Read the model definition and answer for the solid it produces. Units are mm, in the model's axes. Give positions to 0.01 mm unless a question says otherwise; leave off trailing zeros. Write each loop counter-clockwise with the first axis right and the second up, starting at its lowest first coordinate (ties: lowest second). Pieces come first, ordered by that corner, then holes. Notation, with made-up numbers: M 26.5,32.25 L 70.5,32.25 A30 ccw 70.5,70.25 Z; hole C -28.75,77.5 d8. An arc over 180 degrees is marked long. Use a Markdown table: item, result. Add a question column.
Item 1: A cutting plane is placed at A-A on x = 29. Determine the outline of the cut face in (y, z), then the cut area to 3 significant figures.
Item 2: A cutting plane is placed at D-D on z = 14.25. Determine the outline of the cut face in (x, y).
Item 3: Consider probe 1 along X at (y, z) = (66, 2.5); probe 2 along Z at (x, y) = (23.5, 40); probe 3 along X at (y, z) = (47, 3). Determine where each line is inside the solid, lowest interval first. Write a range as [from, to].
Item 4: A cutting plane is placed at C-C on x = 19. Determine the outline of the cut face in (y, z), then the cut area to 3 significant figures.
Item 5: Given P1, Ø1, axis at x = 13.5, y = 51, coming from the +Z side; P2, Ø9.5, axis at x = 21.5, y = 54, coming from the +Z side; P3, Ø8, axis at x = 26, z = 7.5, coming from the -Y side, each flat-ended and moving along its own axis, determine where each tip first touches the part or whether it passes through.
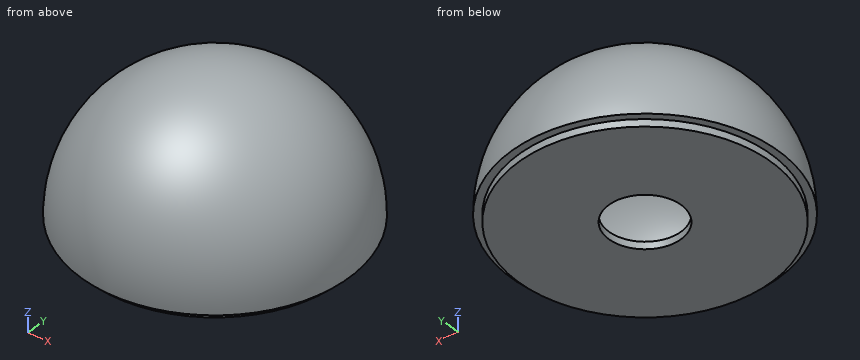
Autodesk Inventor part; units mm, degrees
ref_plane "YZ Plane" through (0, 0, 0) normal (1, 0, 0) x (0, 1, 0)
ref_plane "XZ Plane" through (0, 0, 0) normal (0, 1, 0) x (-1, 0, 0)
ref_plane "XY Plane" through (0, 0, 0) normal (0, 0, 1) x (1, 0, 0)
sketch "Sketch1" plane through (0, 0, 0) normal (0, 0, 1) x (1, 0, 0)
  arc A0 (20.6974, 35.3693) -> (20.6974, 72.3693) centre (20.6974, 53.8693) ccw
  line L0 (20.6974, 72.3693) -> (20.6974, 35.3693)
  circle A1 centre (20.6974, 53.8693) radius 17.5
  point P0 (0, 0)
  dimension "d0" = 37
  dimension "d2" = 35
revolve "Revolution1" add sketch "Sketch1" angle 180 about axis through (20.6974, 72.3693, 0) along (0, -1, 0) picked at (29.7821, 55.9689) contours L0 A1 A0 | L0 A1
shell "Shell2" thickness 3 removed faces 1 at (14.9315, 56.056, 0)
extrude "Extrusion3" add sketch "Sketch1" against normal blind 1 contours A1 L0 | L0 A1
hole "Hole3" at (20.6974, 53.8693, 0) direction (0, 0, -1) diameter 10 depth 1
properties part number "kaca" material "Polycarbonate, Clear"
Filled in:
| question | item | result |
|---|---|---|
| 1 | outline | M 37.34,0 L 38.46,0 L 38.46,-1 L 69.27,-1 L 69.27,0 L 70.4,0 A16.53 ccw Z; hole M 40.78,0 L 66.96,0 A13.09 ccw Z |
| 1 | area | 191 mm² |
| 2 | outline | C 20.7,53.87 d23.6; hole C 20.7,53.87 d12.2 |
| 3 | probe 1 | [6.96, 11.38], [30.02, 34.44] |
| 3 | probe 2 | [-1, 0], [6.33, 11.92] |
| 3 | probe 3 | [3.78, 7.13], [34.26, 37.61] |
| 4 | outline | M 35.45,0 L 36.45,0 L 36.45,-1 L 49.17,-1 L 49.17,0 L 38.46,0 A15.41 cw 69.28,0 L 58.57,0 L 58.57,-1 L 71.29,-1 L 71.29,0 L 72.29,0 A18.42 ccw Z |
| 4 | area | 186 mm² |
| 5 | P1 | z = 17.02 |
| 5 | P2 | z = 18.5 |
| 5 | P3 | y = 36.11 |
